```python
from build123d import *

# Parameters (mm, degrees)
BOSS_EXTRUDE1_DEPTH = 368.3
CUT_EXTRUDE1_REACH  = 154.4
SKETCH2_R           = 9.525
CUT_EXTRUDE2_REACH  = 56.788
SKETCH3_R           = 9.525


with BuildPart() as part:
    # Sketch1 → Boss-Extrude1 (new body, symmetric)
    with BuildSketch(Plane(origin=(0, 0, 0), x_dir=(0, 0, -1), z_dir=(1, 0, 0))):
        with BuildLine():
            Line((-27.3939, -76.2), (-27.3939, 76.2))
            Line((-27.3939, 76.2), (27.3939, 76.2))
            Line((27.3939, 76.2), (27.3939, 73.710744653))
            ThreePointArc((27.3939, 73.710744653), (26.67159656, 71.740607726), (24.84702368, 70.704221901))
            Line((24.84702368, 70.704221901), (-9.926909199, 64.908143628))
            ThreePointArc((-9.926909199, 64.908143628), (-14.488341399, 62.317179067), (-16.2941, 57.391836749))
            Line((-16.2941, 57.391836749), (-16.2941, -57.391836749))
            ThreePointArc((-16.2941, -57.391836749), (-14.488341399, -62.317179067), (-9.926909199, -64.908143628))
            Line((-9.926909199, -64.908143628), (24.84702368, -70.704221901))
            ThreePointArc((24.84702368, -70.704221901), (26.67159656, -71.740607726), (27.3939, -73.710744653))
            Line((27.3939, -73.710744653), (27.3939, -76.2))
            Line((27.3939, -76.2), (-27.3939, -76.2))
        make_face()
    extrude(amount=BOSS_EXTRUDE1_DEPTH, both=True)

    # Sketch2 → Cut-Extrude1 (cut, up to next)
    with BuildSketch(Plane.XZ.offset(76.2), mode=Mode.PRIVATE) as cut_extrude1_sk1:
        with Locations((190.5, -7.5311)):
            Circle(SKETCH2_R)
    cut_extrude1_tool1 = extrude(cut_extrude1_sk1.sketch, amount=-CUT_EXTRUDE1_REACH, mode=Mode.PRIVATE) & part.part
    add(cut_extrude1_tool1.solids().sort_by_distance((190.5, -76.2, -7.5311))[0], mode=Mode.SUBTRACT)
    # Sketch2 → Cut-Extrude1 (cut, up to next)
    with BuildSketch(Plane.XZ.offset(76.2), mode=Mode.PRIVATE) as cut_extrude1_sk2:
        with Locations((-190.5, -7.5311)):
            Circle(SKETCH2_R)
    cut_extrude1_tool2 = extrude(cut_extrude1_sk2.sketch, amount=-CUT_EXTRUDE1_REACH, mode=Mode.PRIVATE) & part.part
    add(cut_extrude1_tool2.solids().sort_by_distance((-190.5, -76.2, -7.5311))[0], mode=Mode.SUBTRACT)
    # Sketch2 → Cut-Extrude1 (cut, up to next)
    with BuildSketch(Plane.XZ.offset(76.2), mode=Mode.PRIVATE) as cut_extrude1_sk3:
        with Locations((330.2, -7.5311)):
            Circle(SKETCH2_R)
    cut_extrude1_tool3 = extrude(cut_extrude1_sk3.sketch, amount=-CUT_EXTRUDE1_REACH, mode=Mode.PRIVATE) & part.part
    add(cut_extrude1_tool3.solids().sort_by_distance((330.2, -76.2, -7.5311))[0], mode=Mode.SUBTRACT)
    # Sketch2 → Cut-Extrude1 (cut, up to next)
    with BuildSketch(Plane.XZ.offset(76.2), mode=Mode.PRIVATE) as cut_extrude1_sk4:
        with Locations((-330.2, -7.5311)):
            Circle(SKETCH2_R)
    cut_extrude1_tool4 = extrude(cut_extrude1_sk4.sketch, amount=-CUT_EXTRUDE1_REACH, mode=Mode.PRIVATE) & part.part
    add(cut_extrude1_tool4.solids().sort_by_distance((-330.2, -76.2, -7.5311))[0], mode=Mode.SUBTRACT)

    # Sketch3 → Cut-Extrude2 (cut, up to next)
    with BuildSketch(Plane.XY.offset(27.3939), mode=Mode.PRIVATE) as cut_extrude2_sk1:
        with Locations((241.3, -30.1625)):
            Circle(SKETCH3_R)
    cut_extrude2_tool1 = extrude(cut_extrude2_sk1.sketch, amount=-CUT_EXTRUDE2_REACH, mode=Mode.PRIVATE) & part.part
    add(cut_extrude2_tool1.solids().sort_by_distance((241.3, -30.1625, 27.3939))[0], mode=Mode.SUBTRACT)
    # Sketch3 → Cut-Extrude2 (cut, up to next)
    with BuildSketch(Plane.XY.offset(27.3939), mode=Mode.PRIVATE) as cut_extrude2_sk2:
        with Locations((-241.3, -30.1625)):
            Circle(SKETCH3_R)
    cut_extrude2_tool2 = extrude(cut_extrude2_sk2.sketch, amount=-CUT_EXTRUDE2_REACH, mode=Mode.PRIVATE) & part.part
    add(cut_extrude2_tool2.solids().sort_by_distance((-241.3, -30.1625, 27.3939))[0], mode=Mode.SUBTRACT)
    # Sketch3 → Cut-Extrude2 (cut, up to next)
    with BuildSketch(Plane.XY.offset(27.3939), mode=Mode.PRIVATE) as cut_extrude2_sk3:
        with Locations((-241.3, 30.1625)):
            Circle(SKETCH3_R)
    cut_extrude2_tool3 = extrude(cut_extrude2_sk3.sketch, amount=-CUT_EXTRUDE2_REACH, mode=Mode.PRIVATE) & part.part
    add(cut_extrude2_tool3.solids().sort_by_distance((-241.3, 30.1625, 27.3939))[0], mode=Mode.SUBTRACT)
    # Sketch3 → Cut-Extrude2 (cut, up to next)
    with BuildSketch(Plane.XY.offset(27.3939), mode=Mode.PRIVATE) as cut_extrude2_sk4:
        with Locations((241.3, 30.1625)):
            Circle(SKETCH3_R)
    cut_extrude2_tool4 = extrude(cut_extrude2_sk4.sketch, amount=-CUT_EXTRUDE2_REACH, mode=Mode.PRIVATE) & part.part
    add(cut_extrude2_tool4.solids().sort_by_distance((241.3, 30.1625, 27.3939))[0], mode=Mode.SUBTRACT)


solid = part.part
```
Here's how the part is built. I have some questions about the finished solid (model axes, mm). A direction names the side the tool comes from. Round coordinates to 2 decimals unless told otherwise and drop trailing zeros. Loops run counter-clockwise (first coordinate to the right, second up) from the corner with the lowest first, then second, coordinate; pieces in that order, holes last. Notation, with made-up numbers: (32.25, -7) -> (68.25, -7) arc R20 cw to (68.25, 14) -> close; hole circle Ø6 at (37.25, -9.5). An arc over 180 degrees is marked (long way). Answer as CSV lines item,"result".
1. If we section it at D-D on x = 330.2: Please give me the cut outline in (y, z).
Final values:
outline,"(-76.2, -27.39) -> (-73.71, -27.39) arc R3.05 ccw to (-70.7, -24.85) -> (-69.41, -17.06) -> (-76.2, -17.06) -> close; (-76.2, 1.99) -> (-66.23, 1.99) -> (-64.91, 9.93) arc R7.62 cw to (-57.39, 16.29) -> (57.39, 16.29) arc R7.62 cw to (64.91, 9.93) -> (70.7, -24.85) arc R3.05 ccw to (73.71, -27.39) -> (76.2, -27.39) -> (76.2, 27.39) -> (-76.2, 27.39) -> close"
2. If we section it at A-A on x = 241.3: Please give me the cut outline in (y, z), plus the area to 3 significant figures.
Final values:
outline,"(-76.2, -27.39) -> (-73.71, -27.39) arc R3.05 ccw to (-70.7, -24.85) -> (-64.91, 9.93) arc R7.62 cw to (-57.39, 16.29) -> (-39.69, 16.29) -> (-39.69, 27.39) -> (-76.2, 27.39) -> close; (-20.64, 16.29) -> (20.64, 16.29) -> (20.64, 27.39) -> (-20.64, 27.39) -> close; (39.69, 16.29) -> (57.39, 16.29) arc R7.62 cw to (64.91, 9.93) -> (70.7, -24.85) arc R3.05 ccw to (73.71, -27.39) -> (76.2, -27.39) -> (76.2, 27.39) -> (39.69, 27.39) -> close"
area,"2,040 mm^2"
3. If I drill on L1, parallel to Y at x = 241.3, z = 23.25; L2, parallel to Z at x = 190.5, y = -74; L3, parallel to Y at x = 19.5, z = 10, over which ranges is the centre line in solid material (lowest first)?
Final values:
L1,"y = -76.2 to -39.69, -20.64 to 20.64, 39.69 to 76.2"
L2,"z = -27.39 to -17.06, 1.99 to 27.39"
L3,"y = -76.2 to -64.9, 64.9 to 76.2"
4. For pin 1 (6 mm diameter, centred on x = 143, y = -29.5, fed in from -Z); pin 2 (17 mm diameter, centred on x = 190.5, z = -7.53, fed in from -Y); pin 3 (15 mm diameter, centred on x = -330.2, z = -7.53, fed in from -Y), each with a flat end and sliding along its axis, tell me the tip position at first contact or that it passes through.
Final values:
pin 1,"stops at z = 16.29"
pin 2,"stops at y = 66.4"
pin 3,"stops at y = 66.57"
5. Which directions (+Z, -Z, +X, -X, +Y, -Y) give clear straight access to the entire face, cutting with the end or side of a thin tool? Please do faces 1 (the face through (5, 1, 16.294)), 2 (the face through (189.26, -72.393, 1.913)), 3 (the face through (5, -76.2, 0)).
Final values:
face 1,"-Z, +X, -X"
face 2,"-Y"
face 3,"+Z, -Z, +X, -X, -Y"
6. If we section it at B-B on x = -51: Please give me the cut outline in (y, z), plus the area to 3 significant figures.
Final values:
outline,"(-76.2, -27.39) -> (-73.71, -27.39) arc R3.05 ccw to (-70.7, -24.85) -> (-64.91, 9.93) arc R7.62 cw to (-57.39, 16.29) -> (57.39, 16.29) arc R7.62 cw to (64.91, 9.93) -> (70.7, -24.85) arc R3.05 ccw to (73.71, -27.39) -> (76.2, -27.39) -> (76.2, 27.39) -> (-76.2, 27.39) -> close"
area,"2,470 mm^2"
7. If we section it at C-C on y = -0.5: Please give me the cut outline in (x, z).
Final values:
outline,"(-368.3, 16.29) -> (368.3, 16.29) -> (368.3, 27.39) -> (-368.3, 27.39) -> close"
8. Thinking about a two-plate mould opening in Z: for faces 4 (the face through (-331.44, -72.393, 1.913)), 5 (the face through (231.784, 30.581, 21.922)), 6 (the face through (5, -1, 27.394)), which applies, released by +Z, released by -Z, zero draft, split by the parting line, or undercut?
Final values:
face 4,"undercut"
face 5,"zero draft"
face 6,"released by +Z"
